from build123d import *

# Parameters (mm, degrees)
SKETCH1_R           = 7.5
SKETCH1_R_2         = 16
BOSS_EXTRUDE1_DEPTH = 15


with BuildPart() as part:
    # Sketch1 → Boss-Extrude1 (new body)
    with BuildSketch(Plane.XY):
        with BuildLine():
            Line((5, 49.282196187), (-5, 49.282196187))
            Line((-5, 49.282196187), (-5, 57.282196187))
            ThreePointArc((-5, 57.282196187), (-49.796460718, 28.75), (-52.107837082, -24.310971075))
            Line((-52.107837082, -24.310971075), (-45.179633852, -20.310971075))
            Line((-45.179633852, -20.310971075), (-40.179633852, -28.971225112))
            Line((-40.179633852, -28.971225112), (-47.107837082, -32.971225112))
            ThreePointArc((-47.107837082, -32.971225112), (0, -57.5), (47.107837082, -32.971225112))
            Line((47.107837082, -32.971225112), (40.179633852, -28.971225112))
            Line((40.179633852, -28.971225112), (45.179633852, -20.310971075))
            Line((45.179633852, -20.310971075), (52.107837082, -24.310971075))
            ThreePointArc((52.107837082, -24.310971075), (56.135775724, -12.450890887), (57.5, 0))
            ThreePointArc((57.5, 0), (42.389562395, 38.85067567), (5, 57.282196187))
            Line((5, 57.282196187), (5, 49.282196187))
        make_face()
        with Locations((0, -40)):
            Circle(SKETCH1_R, mode=Mode.SUBTRACT)
        with Locations((-34.641016151, 20)):
            Circle(SKETCH1_R, mode=Mode.SUBTRACT)
        Circle(SKETCH1_R_2, mode=Mode.SUBTRACT)
        with Locations((34.641016151, 20)):
            Circle(SKETCH1_R, mode=Mode.SUBTRACT)
    extrude(amount=BOSS_EXTRUDE1_DEPTH)


solid = part.part
The model under review builds one solid part; all positions refer to its coordinate system, in mm. A direction names the side the tool comes from. Coordinates: 2 decimals unless noted, no trailing zeros. Loops run counter-clockwise (first coordinate to the right, second up) from the corner with the lowest first, then second, coordinate; pieces in that order, holes last. Notation, with made-up numbers: M 81,55 L 99,55 A37 ccw 99,94 Z; hole C 40.5,79 d1. An arc over 180 degrees is marked long. Put each result on its own line as item: value. Start each with the question number.
Q1. Wall thickness on line 1 (Y direction, x = 0, z = 5.75); line 2 (Y direction, x = 6, z = 13); line 3 (X direction, y = 0.5, z = 2): over which ranges is each line inside the solid? List them lowest first.
Q2. The part is to be moulded in two halves that separate along Y. For faces 1 (the flat face through (0, 49.282, 7)), 2 (the flat face through (12, -12, 15)), 3 (the flat face through (-48.692, -22.339, 7.395)), 4 (the cylindrical face through (-3.47, -15.62, 7.4)), say which applies: +Y half, -Y half, draft (parallel to the pull), parting line (faces both ways), or undercut.
Q3. For faces 5 (the flat face through (-43.595, -30.943, 7.395)), 6 (the flat face through (-5, 53, 7)), 7 (the flat face through (43.69, -31, 7.4)), 8 (the flat face through (42.645, -24.702, 7.395)), list the 3-axis set-ups (+Z, -Z, +X, -X, +Y, -Y) from which the entire face can be reached by the end or side of a thin tool; tool diameter is ignored.
Q4. Add section C-C (z = 3.75). Write out the cut boundary in (x, y).
Q5. Add section A-A (x = 0). Write out the cut boundary in (y, z), and give its area (3 significant figures).
Q6. Add section B-B (y = -23). Write out the cut boundary in (x, z), and give its area (3 significant figures).
Q7. Add section D-D (y = -40). Write out the cut boundary in (x, z), and give its area (3 significant figures).
Q8. Clearance check with flat-ended pins moving along their axes: pin 1 (3 mm diameter, centred on x = 23.5, z = 11, fed in from -Y); pin 2 (6 mm diameter, centred on y = 39, z = 12.5, fed in from +X); pin 3 (6.5 mm diameter, centred on y = 52, z = 6, fed in from +X); pin 4 (5 mm diameter, centred on x = -29, y = -27.5, fed in from -Z). State where each tip first meets the part, or that it passes through.
Answers:
1. line 1: y = -57.5 to -47.5, -32.5 to -16, 16 to 49.28
1. line 2: y = -57.19 to -44.5, -35.5 to -14.83, 14.83 to 57.19
1. line 3: x = -57.5 to -15.99, 15.99 to 57.5
2. face 1: +Y half
2. face 2: draft
2. face 3: undercut
2. face 4: undercut
3. face 5: +Z, -Z, -X
3. face 6: +Z, -Z, +Y
3. face 7: +Z, -Z, +X
3. face 8: +Z, -Z
4. outline: M -52.11,-24.31 L -45.18,-20.31 L -40.18,-28.97 L -47.11,-32.97 A57.5 ccw 47.11,-32.97 L 40.18,-28.97 L 45.18,-20.31 L 52.11,-24.31 A57.5 ccw 5,57.28 L 5,49.28 L -5,49.28 L -5,57.28 A57.5 ccw Z; hole C -34.64,20 d15; hole C 0,0 d32; hole C 0,-40 d15; hole C 34.64,20 d15
5. outline: M -57.5,0 L -47.5,0 L -47.5,15 L -57.5,15 Z; M -32.5,0 L -16,0 L -16,15 L -32.5,15 Z; M 16,0 L 49.28,0 L 49.28,15 L 16,15 Z
5. area: 897 mm^2
6. outline: M -52.7,0 L -49.84,0 L -49.84,15 L -52.7,15 Z; M -43.63,0 L 43.63,0 L 43.63,15 L -43.63,15 Z; M 49.84,0 L 52.7,0 L 52.7,15 L 49.84,15 Z
6. area: 1,390 mm^2
7. outline: M -41.31,0 L -7.5,0 L -7.5,15 L -41.31,15 Z; M 7.5,0 L 41.31,0 L 41.31,15 L 7.5,15 Z
7. area: 1,010 mm^2
8. pin 1: stops at y = -53.12
8. pin 2: stops at x = 44.84
8. pin 3: stops at x = 30.49
8. pin 4: stops at z = 0
